Geometry check sheet. Reference: the model listing, model coordinates, mm. Face numbers are marked on the shaded views. Give positions to 0.01 mm unless a question says otherwise; leave off trailing zeros. Write each loop counter-clockwise with the first axis right and the second up, starting at its lowest first coordinate (ties: lowest second). Pieces come first, ordered by that corner, then holes. Notation, with made-up numbers: (-25, -34) - (16, -34) arc R16 cw to (16, -17) - close; hole circle Ø2 at (0.25, 60). An arc over 180 degrees is marked (long way). Use a Markdown table: item, result.
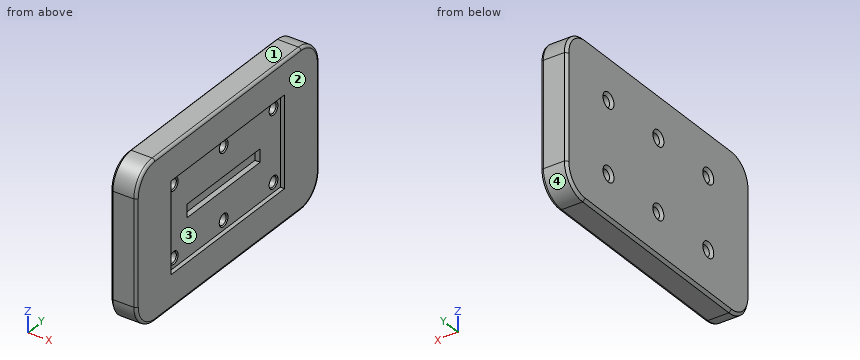
```python
from build123d import *

# Parameters (mm, degrees)
SKETCH1_W           = 60
SKETCH1_H           = 100
BOSS_EXTRUDE1_DEPTH = 10
SKETCH2_W           = 34.6
SKETCH2_H           = 62
CUT_EXTRUDE1_DEPTH  = 1.6
SKETCH3_R           = 2
CUT_EXTRUDE2_DEPTH  = 59.911458987
FILLET1_R           = 10
FILLET2_R           = 1
CHAMFER1_SIZE       = 1
CHAMFER2_SIZE       = 0.4
SKETCH4_W           = 5
SKETCH4_H           = 40
CUT_EXTRUDE3_DEPTH  = 2


with BuildPart() as part:
    # Sketch1 → Boss-Extrude1 (new body)
    with BuildSketch(Plane(origin=(0, 0, 0), x_dir=(0, 0, -1), z_dir=(1, 0, 0))):
        Rectangle(SKETCH1_W, SKETCH1_H)
    extrude(amount=BOSS_EXTRUDE1_DEPTH)

    # Sketch2 → Cut-Extrude1 (cut)
    with BuildSketch(Plane(origin=(10, 0, 0), x_dir=(0, 0, -1), z_dir=(1, 0, 0))):
        Rectangle(SKETCH2_W, SKETCH2_H)
    extrude(amount=-CUT_EXTRUDE1_DEPTH, mode=Mode.SUBTRACT)

    # Sketch3 → Cut-Extrude2 (cut, through all)
    with BuildSketch(Plane(origin=(8.4, 0, 0), x_dir=(0, 0, -1), z_dir=(1, 0, 0))):
        with Locations((-13.6, 27.3)):
            Circle(SKETCH3_R)
        with Locations((13.6, 27.3)):
            Circle(SKETCH3_R)
        with Locations((-13.6, 0)):
            Circle(SKETCH3_R)
        with Locations((13.6, 0)):
            Circle(SKETCH3_R)
        with Locations((-13.6, -27.3)):
            Circle(SKETCH3_R)
        with Locations((13.6, -27.3)):
            Circle(SKETCH3_R)
    extrude(amount=-CUT_EXTRUDE2_DEPTH, mode=Mode.SUBTRACT)

    # Fillet1
    fillet1_edges = [part.edges().sort_by_distance(p)[0] for p in [
        (5, -50, -30),
        (5, -50, 30),
        (5, 50, 30),
        (5, 50, -30),
    ]]
    fillet(fillet1_edges, radius=FILLET1_R)

    # Fillet2
    fillet2_edges = [part.edges().sort_by_distance(p)[0] for p in [
        (10, -50, 0),
        (10, 0, 30),
        (10, 0, -30),
        (10, 50, 0),
        (10, -47.071067812, -27.071067812),
        (10, 47.071067812, -27.071067812),
        (10, 47.071067812, 27.071067812),
        (10, -47.071067812, 27.071067812),
    ]]
    fillet(fillet2_edges, radius=FILLET2_R)

    # Chamfer1
    chamfer1_edges = [part.edges().sort_by_distance(p)[0] for p in [
        (0, -27.3, 15.6),
        (0, 0, -11.6),
        (0, 0, 15.6),
        (0, 27.3, -11.6),
        (0, -27.3, -11.6),
        (0, 27.3, 15.6),
        (0, -50, 0),
        (0, 0, -30),
        (0, 0, 30),
        (0, 50, 0),
        (0, -47.071067812, -27.071067812),
        (0, 47.071067812, -27.071067812),
        (0, 47.071067812, 27.071067812),
        (0, -47.071067812, 27.071067812),
    ]]
    chamfer(chamfer1_edges, length=CHAMFER1_SIZE)

    # Chamfer2
    chamfer2_edges = [part.edges().sort_by_distance(p)[0] for p in [
        (8.4, -27.3, 15.6),
        (8.4, 0, -11.6),
        (8.4, 0, 15.6),
        (8.4, 27.3, -11.6),
        (8.4, -27.3, -11.6),
        (8.4, 27.3, 15.6),
    ]]
    chamfer(chamfer2_edges, length=CHAMFER2_SIZE)

    # Sketch4 → Cut-Extrude3 (cut)
    with BuildSketch(Plane(origin=(8.4, 0, 0), x_dir=(0, 0, -1), z_dir=(1, 0, 0))):
        Rectangle(SKETCH4_W, SKETCH4_H)
    extrude(amount=-CUT_EXTRUDE3_DEPTH, mode=Mode.SUBTRACT)


solid = part.part
```
1) Material ranges on L1, parallel to Y at x = 5.25, z = 13.6; L2, parallel to Y at x = 8.25, z = 1; L3, parallel to Z at x = 7.75, y = 18.5, recorded low to high. Write a range as from..to.
Working result:
| item | result |
|---|---|
| L1 | y = -50..-29.3, -25.3..-2, 2..25.3, 29.3..50 |
| L2 | y = -50..-20, 20..50 |
| L3 | z = -30..-2.5, 2.5..30 |
2) Depth check by flat-ended pin: P1, Ø3, axis at y = 27.3, z = 13.6, coming from the -X side; P2, Ø17.5, axis at y = 11, z = 6.5, coming from the +X side; P3, Ø0.8, axis at x = 9.5, z = -4.5, coming from the +Y side (3 decimals); P4, Ø2.5, axis at y = 2, z = 1, coming from the +X side. Enter the tip coordinate at first touch or a pass-through.
Working result:
| item | result |
|---|---|
| P1 | passes through |
| P2 | stops at x = 8.4 |
| P3 | stops at y = 49.995 |
| P4 | stops at x = 6.4 |
3) Section check D-D on z = 13.6. Count the separate pieces of the cut face and the enclosed holes in it, then the cut area to 3 significant figures.
Working result:
| item | result |
|---|---|
| separate pieces | 4 |
| enclosed holes | 0 |
| area | 795 mm² |
4) Mould release check, pull along Z, two halves, no side actions. Record for the marked faces 1, 2, 3 and 4: pulls with the +Z half, pulls with the -Z half, needs draft (parallel to the pull), parting line crosses it, or undercut.
Working result:
| item | result |
|---|---|
| face 1 | pulls with the +Z half |
| face 2 | needs draft |
| face 3 | undercut |
| face 4 | pulls with the -Z half |
5) Section check A-A on y = -27.3. Record the boundary of the cut face in (x, z), then the cut area to 3 significant figures.
Working result:
| item | result |
|---|---|
| outline | (0, -29) - (1, -30) - (9, -30) arc R1 ccw to (10, -29) - (10, -17.3) - (8.4, -17.3) - (8.4, -16) - (8, -15.6) - (1, -15.6) - (0, -16.6) - close; (0, -10.6) - (1, -11.6) - (8, -11.6) - (8.4, -11.2) - (8.4, 11.2) - (8, 11.6) - (1, 11.6) - (0, 10.6) - close; (0, 16.6) - (1, 15.6) - (8, 15.6) - (8.4, 16) - (8.4, 17.3) - (10, 17.3) - (10, 29) arc R1 ccw to (9, 30) - (1, 30) - (0, 29) - close |
| area | 474 mm² |
6) Section check C-C on y = -5. Record the boundary of the cut face in (x, z).
Working result:
| item | result |
|---|---|
| outline | (0, -29) - (1, -30) - (9, -30) arc R1 ccw to (10, -29) - (10, -17.3) - (8.4, -17.3) - (8.4, -2.5) - (6.4, -2.5) - (6.4, 2.5) - (8.4, 2.5) - (8.4, 17.3) - (10, 17.3) - (10, 29) arc R1 ccw to (9, 30) - (1, 30) - (0, 29) - close |
7) Section check B-B on x = 3.75. Record the boundary of the cut face in (y, z), then the cut area to 3 significant figures.
Working result:
| item | result |
|---|---|
| outline | (-50, -20) arc R10 ccw to (-40, -30) - (40, -30) arc R10 ccw to (50, -20) - (50, 20) arc R10 ccw to (40, 30) - (-40, 30) arc R10 ccw to (-50, 20) - close; hole circle Ø4 at (-27.3, -13.6); hole circle Ø4 at (-27.3, 13.6); hole circle Ø4 at (0, -13.6); hole circle Ø4 at (0, 13.6); hole circle Ø4 at (27.3, -13.6); hole circle Ø4 at (27.3, 13.6) |
| area | 5,840 mm² |
